```python
from build123d import *

# Parameters (mm, degrees)
SKETCH1_W           = 120
SKETCH1_H           = 310
BOSS_EXTRUDE4_DEPTH = 90
SHELL2_T            = -5
SKETCH2_R           = 7.499675099
CUT_EXTRUDE1_DEPTH  = 10
SKETCH3_W           = 120
SKETCH3_H           = 20
BOSS_EXTRUDE5_DEPTH = 25
SKETCH4_R           = 2.5
CUT_EXTRUDE2_DEPTH  = 20
FILLET1_R           = 5


with BuildPart() as part:
    # Sketch1 → Boss-Extrude4 (new body)
    with BuildSketch(Plane(origin=(0, 0, 0), x_dir=(1, 0, 0), z_dir=(0, 1, 0))):
        with Locations((240, 0)):
            Rectangle(SKETCH1_W, SKETCH1_H)
    extrude(amount=BOSS_EXTRUDE4_DEPTH)

    # Shell2
    shell2_openings = [part.faces().sort_by_distance(p)[0] for p in [
        (240, 90, 0),
    ]]
    offset(amount=SHELL2_T, openings=shell2_openings, kind=Kind.INTERSECTION)

    # Sketch2 → Cut-Extrude1 (cut)
    with BuildSketch(Plane.ZY.offset(-180)):
        with Locations((-125, 40)):
            Circle(SKETCH2_R)
        with Locations((125, 40)):
            Circle(SKETCH2_R)
    extrude(amount=-CUT_EXTRUDE1_DEPTH, mode=Mode.SUBTRACT)

    # Sketch3 → Boss-Extrude5 (add)
    with BuildSketch(Plane.XY.offset(180)):
        with Locations((240, 45)):
            Rectangle(SKETCH3_W, SKETCH3_H)
    boss_extrude5 = extrude(amount=-BOSS_EXTRUDE5_DEPTH)

    # Mirror1: Boss-Extrude5 across plane
    add(boss_extrude5.mirror(Plane.XY))

    # Sketch4 → Cut-Extrude2 (cut)
    with BuildSketch(Plane(origin=(180, 0, 0), x_dir=(0, 0, -1), z_dir=(1, 0, 0))):
        with Locations((-170, 45)):
            Circle(SKETCH4_R)
        with Locations((170, 45)):
            Circle(SKETCH4_R)
    extrude(amount=CUT_EXTRUDE2_DEPTH, mode=Mode.SUBTRACT)

    # Fillet1
    fillet1_edges = [part.edges().sort_by_distance(p)[0] for p in [
        (300, 17.5, 155),
        (180, 17.5, 155),
        (240, 55, 155),
        (240, 35, 155),
        (180, 55, 167.5),
        (180, 35, 167.5),
        (240, 55, 180),
        (240, 35, 180),
        (300, 55, 167.5),
        (300, 35, 167.5),
        (180, 17.5, -155),
        (300, 17.5, -155),
        (240, 35, -155),
        (240, 55, -155),
        (180, 35, -167.5),
        (240, 35, -180),
        (180, 55, -167.5),
        (300, 35, -167.5),
        (300, 55, -167.5),
        (240, 55, -180),
        (180, 72.5, -155),
        (300, 72.5, -155),
        (300, 72.5, 155),
        (180, 72.5, 155),
    ]]
    fillet(fillet1_edges, radius=FILLET1_R)


solid = part.part
```
The listing builds one solid part. Answer for the finished solid, in the listing's coordinates (mm). A direction names the side the tool comes from. Give positions to 0.01 mm unless a question says otherwise; leave off trailing zeros. Write each loop counter-clockwise with the first axis right and the second up, starting at its lowest first coordinate (ties: lowest second). Pieces come first, ordered by that corner, then holes. Notation, with made-up numbers: (-30.75, 13) - (-20.75, 13) arc R18 cw to (-20.75, 30) - close; hole circle Ø10 at (-1.5, 58.25). An arc over 180 degrees is marked (long way). Use one line per item in the form item = value. Start each with the question number.
1) Consider line 1 along Y through (x, z) = (192, -170); line 2 along Z through (x, y) = (229.5, 59.5); line 3 along X through (y, z) = (49, 58). Determine where each line is inside the solid, lowest interval first. Write a range as from..to.
2) Find section B-B on y = 80. Determine the outline of the cut face in (x, z).
3) Find section D-D on z = -8.5. Determine the outline of the cut face in (x, y), plus the area to 3 significant figures.
4) A tool of negligible diameter and unlimited length cuts with its end or side. For faces 4 (the face through (239, 35, 168)), 5 (the face through (295, 47, 2)), 6 (the face through (182.465, 40.33, -132.492)), 7 (the face through (239, 55, 168)), from which of +Z, -Z, +X, -X, +Y, -Y can it reach the whole face along a straight path? Write none if from no direction.
5) The mould has two halves that part along X. Classify faces 1 (the face through (239, 15, -155)), 2 (the face through (300, 44, 3)), 3 (the face through (239, 47, -150)): pulls with the +X half, pulls with the -X half, needs draft (parallel to the pull), parting line crosses it, or undercut.
6) Find section C-C on x = 251.5. Determine the outline of the cut face in (y, z), plus the area to 3 significant figures.
7) Flat-ended cylindrical pins translate along their axes: pin 1 Ø7.5 at (x, z) = (236.5, -167.5) entering from +Y; pin 2 Ø24 at (x, y) = (216.5, 11.5) entering from -Z; pin 3 Ø9 at (x, y) = (234, 71) entering from +Z. Find the tip coordinate at first contact, or state that the pin passes through.
8) Find section A-A on z = -125. Determine the outline of the cut face in (x, y), plus the area to 4 significant figures.
Geometry results:
q1.line_1 = 35..42.5, 47.5..55
q1.line_2 = -155.03..-150, 150..155.03
q1.line_3 = 180..185, 295..300
q2.outline = (180, -150) arc R5 ccw to (185, -155) - (295, -155) arc R5 ccw to (300, -150) - (300, 150) arc R5 ccw to (295, 155) - (185, 155) arc R5 ccw to (180, 150) - close; hole (185, -150) - (295, -150) - (295, 150) - (185, 150) - close
q3.outline = (180, 0) - (300, 0) - (300, 90) - (295, 90) - (295, 5) - (185, 5) - (185, 90) - (180, 90) - close
q3.area = 1,450 mm2
q4.face_4 = +Z, +X, -X, -Y
q4.face_5 = +Y
q4.face_6 = -X
q4.face_7 = +Z, +X, -X, +Y
q5.face_1 = needs draft
q5.face_2 = pulls with the +X half
q5.face_3 = undercut
q6.outline = (0, -155) - (30, -155) arc R5 cw to (35, -160) - (35, -175) arc R5 ccw to (40, -180) - (50, -180) arc R5 ccw to (55, -175) - (55, -160) arc R5 cw to (60, -155) - (90, -155) - (90, -150) - (5, -150) - (5, 150) - (90, 150) - (90, 155) - (60, 155) arc R5 cw to (55, 160) - (55, 175) arc R5 ccw to (50, 180) - (40, 180) arc R5 ccw to (35, 175) - (35, 160) arc R5 cw to (30, 155) - (0, 155) - close
q6.area = 3,400 mm2
q7.pin_1 = 55
q7.pin_2 = -155
q7.pin_3 = 155
q8.outline = (180, 0) - (300, 0) - (300, 90) - (295, 90) - (295, 5) - (185, 5) - (185, 32.5) - (180, 32.5) - close; (180, 47.5) - (185, 47.5) - (185, 90) - (180, 90) - close
q8.area = 1,375 mm2
